Geometry: final body of the model. Coordinates: model frame, mm. A direction names the side the tool comes from. Give positions to 0.01 mm unless a question says otherwise; leave off trailing zeros. Order: outer loops, then holes, each group sorted by start corner. A loop starts at its lowest first (then second) coordinate and runs counter-clockwise, first axis right, second up. Notation, with made-up numbers: (-21.75, -10.5) -> (7.25, -10.5) arc R19 ccw to (7.25, 11.5) -> close; hole circle Ø8 at (-4.5, 65). An arc over 180 degrees is marked (long way). Write item = value, one per line.
```python
from build123d import *

# Parameters (mm, degrees)
CROQUIS2_W              = 75
CROQUIS2_H              = 100
SALIENTE_EXTRUIR1_DEPTH = 40
CROQUIS3_W              = 75
CROQUIS3_H              = 5
SALIENTE_EXTRUIR2_DEPTH = 5
CROQUIS4_R              = 10
CROQUIS4_R_2            = 6
SALIENTE_EXTRUIR7_DEPTH = 10
CROQUIS9_R              = 6
SALIENTE_EXTRUIR8_DEPTH = 30


with BuildPart() as part:
    # Croquis2 → Saliente-Extruir1 (new body)
    with BuildSketch(Plane(origin=(0, 0, 0), x_dir=(1, 0, 0), z_dir=(0, 1, 0))):
        Rectangle(CROQUIS2_W, CROQUIS2_H)
    extrude(amount=SALIENTE_EXTRUIR1_DEPTH)

    # Croquis3 → Saliente-Extruir2 (add)
    with BuildSketch(Plane.XZ):
        with Locations((0, 25)):
            Rectangle(CROQUIS3_W, CROQUIS3_H)
        with Locations((0, -25)):
            Rectangle(CROQUIS3_W, CROQUIS3_H)
    extrude(amount=SALIENTE_EXTRUIR2_DEPTH)

    # Croquis4 → Saliente-Extruir7 (add)
    # profile 1 of 4: a face of its own
    with BuildSketch(Plane(origin=(0, 40, 0), x_dir=(1, 0, 0), z_dir=(0, 1, 0))):
        with Locations(Location((-26.5, 39, 0), (0, 0, 90))):
            Circle(CROQUIS4_R)
        with Locations(Location((-26.5, 39, 0), (0, 0, 270))):
            Circle(CROQUIS4_R_2, mode=Mode.SUBTRACT)
    # profile 2 of 4: a face of its own
    with BuildSketch(Plane(origin=(0, 40, 0), x_dir=(1, 0, 0), z_dir=(0, 1, 0))):
        with Locations(Location((26.5, 39, 0), (0, 0, 90))):
            Circle(CROQUIS4_R)
        with Locations(Location((26.5, 39, 0), (0, 0, 90))):
            Circle(CROQUIS4_R_2, mode=Mode.SUBTRACT)
    # profile 3 of 4: a face of its own
    with BuildSketch(Plane(origin=(0, 40, 0), x_dir=(1, 0, 0), z_dir=(0, 1, 0))):
        with Locations(Location((26.5, -39, 0), (0, 0, 90))):
            Circle(CROQUIS4_R)
        with Locations(Location((26.5, -39, 0), (0, 0, 270))):
            Circle(CROQUIS4_R_2, mode=Mode.SUBTRACT)
    # profile 4 of 4: a face of its own
    with BuildSketch(Plane(origin=(0, 40, 0), x_dir=(1, 0, 0), z_dir=(0, 1, 0))):
        with Locations(Location((-26.5, -39, 0), (0, 0, 90))):
            Circle(CROQUIS4_R)
        with Locations(Location((-26.5, -39, 0), (0, 0, 90))):
            Circle(CROQUIS4_R_2, mode=Mode.SUBTRACT)
    extrude(amount=SALIENTE_EXTRUIR7_DEPTH)

    # Croquis9 → Saliente-Extruir8 (add)
    with BuildSketch(Plane(origin=(0, 40, 0), x_dir=(1, 0, 0), z_dir=(0, 1, 0))):
        with Locations(Location((-26.5, -39, 0), (0, 0, 90))):
            Circle(CROQUIS9_R)
        with Locations(Location((-26.5, 39, 0), (0, 0, 90))):
            Circle(CROQUIS9_R)
        with Locations(Location((26.5, -39, 0), (0, 0, 90))):
            Circle(CROQUIS9_R)
        with Locations(Location((26.5, 39, 0), (0, 0, 90))):
            Circle(CROQUIS9_R)
    extrude(amount=SALIENTE_EXTRUIR8_DEPTH)


solid = part.part
```
1) Line query: line 1 (Z direction, x = -25, y = -2); line 2 (Y direction, x = -17, z = -14.5); line 3 (Y direction, x = -33, z = 32). Output: solid intervals per line, ascending. Write a range as from..to.
Check sheet entries:
line_1 = -27.5..-22.5, 22.5..27.5
line_2 = 0..40
line_3 = 0..50
2) Mould query, pull axis Z, two halves, no side actions, for faces 5 (the face through (-26.94, 44.93, 48.99)), 6 (the face through (-1, 20, 50)), 7 (the face through (-1, 20, -50)), 8 (the face through (-1, -5, -25)). Classes: +Z half, -Z half, draft (parallel to the pull), parting line (faces both ways), or undercut.
Check sheet entries:
face_5 = undercut
face_6 = +Z half
face_7 = -Z half
face_8 = draft
3) Section query D-D (x = 26.5). Output: boundary loops of the cut face in (y, z), plus the area to 3 significant figures.
Check sheet entries:
outline = (-5, -27.5) -> (0, -27.5) -> (0, -50) -> (40, -50) -> (40, -49) -> (50, -49) -> (50, -45) -> (70, -45) -> (70, -33) -> (50, -33) -> (50, -29) -> (40, -29) -> (40, 29) -> (50, 29) -> (50, 33) -> (70, 33) -> (70, 45) -> (50, 45) -> (50, 49) -> (40, 49) -> (40, 50) -> (0, 50) -> (0, 27.5) -> (-5, 27.5) -> (-5, 22.5) -> (0, 22.5) -> (0, -22.5) -> (-5, -22.5) -> close
area = 4,930 mm²
4) Section query B-B (y = 45.5). Output: boundary loops of the cut face in (x, z), plus the area to 3 significant figures.
Check sheet entries:
outline = circle Ø20 at (-26.5, -39); circle Ø20 at (-26.5, 39); circle Ø20 at (26.5, -39); circle Ø20 at (26.5, 39)
area = 1,260 mm²
5) First-contact query: P1, Ø2.5, axis at x = 5.5, y = -2.5, coming from the -Z side; P2, Ø7, axis at x = 6.5, z = 33.5, coming from the -Y side; P3, Ø5, axis at x = -16, z = -6, coming from the +Y side; P4, Ø6, axis at x = 5, y = 45.5, coming from the +Z side. Flat tips, straight axial feed; report the tip coordinate or a pass-through.
Check sheet entries:
P1 = -27.5
P2 = 0
P3 = 40
P4 = through
6) Reachability of faces 1 (the face through (-1, -2, 27.5)), 2 (the face through (-27, 70, 39)), 3 (the face through (-1, -2, 22.5)), 4 (the face through (-1, 40, -1)) from +Z, -Z, +X, -X, +Y, -Y: full face, straight path, thin tool, end or side. Return the list, or none.
Check sheet entries:
face_1 = +Z, +X, -X, -Y
face_2 = +Z, -Z, +X, -X, +Y
face_3 = +X, -X, -Y
face_4 = +Y
7) Section query A-A (z = 39). Output: boundary loops of the cut face in (x, y), plus the area to 3 significant figures.
Check sheet entries:
outline = (-37.5, 0) -> (37.5, 0) -> (37.5, 40) -> (36.5, 40) -> (36.5, 50) -> (32.5, 50) -> (32.5, 70) -> (20.5, 70) -> (20.5, 50) -> (16.5, 50) -> (16.5, 40) -> (-16.5, 40) -> (-16.5, 50) -> (-20.5, 50) -> (-20.5, 70) -> (-32.5, 70) -> (-32.5, 50) -> (-36.5, 50) -> (-36.5, 40) -> (-37.5, 40) -> close
area = 3,880 mm²
8) Section query C-C (x = -10). Output: boundary loops of the cut face in (y, z).
Check sheet entries:
outline = (-5, -27.5) -> (0, -27.5) -> (0, -50) -> (40, -50) -> (40, 50) -> (0, 50) -> (0, 27.5) -> (-5, 27.5) -> (-5, 22.5) -> (0, 22.5) -> (0, -22.5) -> (-5, -22.5) -> close
